```python
from build123d import *

# Parameters (mm, degrees)
BOSS_EXTRUDE2_DEPTH             = 400
SHELL3_T                        = -3
FILLET2_R                       = 50
FILLET3_R                       = 50
BOSS_EXTRUDE3_REACH             = 1052
SKETCH3_W                       = 40
SKETCH3_H                       = 40
BOSS_EXTRUDE3_DIRECTION_2_DEPTH = 19.71
SKETCH4_R                       = 7.5
CUT_EXTRUDE1_DEPTH              = 20


with BuildPart() as part:
    # Sketch2 → Boss-Extrude2 (new body)
    with BuildSketch(Plane.XY):
        Polygon((0, 400), (0, 0), (-400, 107.179676972), (-400, 207.179676972), align=None)
    extrude(amount=BOSS_EXTRUDE2_DEPTH)

    # Shell3
    shell3_openings = [part.faces().sort_by_distance(p)[0] for p in [
        (-400, 157.179676972, 200),
        (-200, 303.589838486, 200),
    ]]
    offset(amount=SHELL3_T, openings=shell3_openings, kind=Kind.INTERSECTION)

    # Fillet2
    fillet2_edges = [part.edges().sort_by_distance(p)[0] for p in [
        (-400, 207.179676972, 398.5),
    ]]
    fillet(fillet2_edges, radius=FILLET2_R)

    # Fillet3
    fillet3_edges = [part.edges().sort_by_distance(p)[0] for p in [
        (-400, 207.179676972, 1.5),
    ]]
    fillet(fillet3_edges, radius=FILLET3_R)

    # Sketch3 → Boss-Extrude3 (add, up to next)
    with BuildSketch(Plane(origin=(0, -650, 0), x_dir=(1, 0, 0), z_dir=(0, 1, 0)), mode=Mode.PRIVATE) as boss_extrude3_sk1:
        with Locations((-83, -60)):
            Rectangle(SKETCH3_W, SKETCH3_H)
    boss_extrude3_tool1 = extrude(boss_extrude3_sk1.sketch, amount=BOSS_EXTRUDE3_REACH, mode=Mode.PRIVATE) - part.part
    add(boss_extrude3_tool1.solids().sort_by_distance((-83, -650, 60))[0])
    # Sketch3 → Boss-Extrude3 (add, up to next)
    with BuildSketch(Plane(origin=(0, -650, 0), x_dir=(1, 0, 0), z_dir=(0, 1, 0)), mode=Mode.PRIVATE) as boss_extrude3_sk2:
        with Locations((-320, -60)):
            Rectangle(SKETCH3_W, SKETCH3_H)
    boss_extrude3_tool2 = extrude(boss_extrude3_sk2.sketch, amount=BOSS_EXTRUDE3_REACH, mode=Mode.PRIVATE) - part.part
    add(boss_extrude3_tool2.solids().sort_by_distance((-320, -650, 60))[0])
    # Sketch3 → Boss-Extrude3 (add, up to next)
    with BuildSketch(Plane(origin=(0, -650, 0), x_dir=(1, 0, 0), z_dir=(0, 1, 0)), mode=Mode.PRIVATE) as boss_extrude3_sk3:
        with Locations((-83, -340)):
            Rectangle(SKETCH3_W, SKETCH3_H)
    boss_extrude3_tool3 = extrude(boss_extrude3_sk3.sketch, amount=BOSS_EXTRUDE3_REACH, mode=Mode.PRIVATE) - part.part
    add(boss_extrude3_tool3.solids().sort_by_distance((-83, -650, 340))[0])
    # Sketch3 → Boss-Extrude3 (add, up to next)
    with BuildSketch(Plane(origin=(0, -650, 0), x_dir=(1, 0, 0), z_dir=(0, 1, 0)), mode=Mode.PRIVATE) as boss_extrude3_sk4:
        with Locations((-320, -340)):
            Rectangle(SKETCH3_W, SKETCH3_H)
    boss_extrude3_tool4 = extrude(boss_extrude3_sk4.sketch, amount=BOSS_EXTRUDE3_REACH, mode=Mode.PRIVATE) - part.part
    add(boss_extrude3_tool4.solids().sort_by_distance((-320, -650, 340))[0])

    # Sketch3 → Boss-Extrude3 direction 2 (add)
    with BuildSketch(Plane(origin=(0, -650, 0), x_dir=(1, 0, 0), z_dir=(0, 1, 0))):
        with Locations((-83, -60)):
            Rectangle(SKETCH3_W, SKETCH3_H)
        with Locations((-320, -60)):
            Rectangle(SKETCH3_W, SKETCH3_H)
        with Locations((-83, -340)):
            Rectangle(SKETCH3_W, SKETCH3_H)
        with Locations((-320, -340)):
            Rectangle(SKETCH3_W, SKETCH3_H)
    extrude(amount=-BOSS_EXTRUDE3_DIRECTION_2_DEPTH)

    # Sketch4 → Cut-Extrude1 (cut)
    with BuildSketch(Plane.XZ.offset(669.71)):
        with Locations((-320, 340)):
            Circle(SKETCH4_R)
        with Locations((-83, 340)):
            Circle(SKETCH4_R)
        with Locations((-320, 60)):
            Circle(SKETCH4_R)
        with Locations((-83, 60)):
            Circle(SKETCH4_R)
    extrude(amount=-CUT_EXTRUDE1_DEPTH, mode=Mode.SUBTRACT)


solid = part.part
```
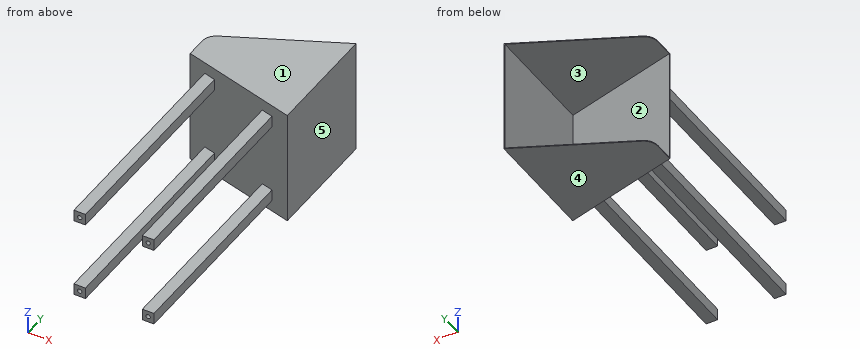
Work out the finished part from the listing and answer in its coordinate system (mm). Face numbers are marked on the shaded views. A direction names the side the tool comes from. Give positions to 0.01 mm unless a question says otherwise; leave off trailing zeros. Loops run counter-clockwise (first coordinate to the right, second up) from the corner with the lowest first, then second, coordinate; pieces in that order, holes last. Notation, with made-up numbers: (-11, 35.25) -> (3, 35.25) arc R16 ccw to (3, 64.25) -> close; hole circle Ø8 at (-34.5, 61). An arc over 180 degrees is marked (long way). Write item = value, one per line. Start each with the question number.
(1) Find section A-A on y = -397.5. Give the vertices of the cut face in (x, z).
(2) Find the intervals of material crossed by probe 1 along Z at (x, y) = (-320, -661); probe 2 along X at (y, z) = (-661.75, 340); probe 3 along X at (y, z) = (-619, 327), in increasing order. Write a range as from..to.
(3) Which of the six approach directions +Z, -Z, +X, -X, +Y, -Y give full straight-line access (tool end or side, diameter ignored) to the marked faces 1 and 2?
(4) The mould has two halves that part along X. Classify the marked faces 3, 4 and 5: +X half, -X half, draft (parallel to the pull), parting line (faces both ways), or undercut.
(5) Find section B-B on y = 149. Give the vertices of the cut face in (x, z).
(6) Given pin 1 Ø20 at (x, y) = (-314.5, -342.5) entering from -Z; pin 2 Ø1.5 at (x, z) = (-331.5, 356) entering from +Y; pin 3 Ø20 at (y, z) = (-246, 68.5) entering from -X, each flat-ended and moving along its own axis, determine where each tip first touches the part or whether it passes through.
(7) Find section C-C on x = -351. Give the vertices of the cut face in (y, z), and give its area (3 significant figures).
From the geometry:
q1.outline = (-340, 40) -> (-300, 40) -> (-300, 80) -> (-340, 80) -> close; (-340, 320) -> (-300, 320) -> (-300, 360) -> (-340, 360) -> close; (-103, 40) -> (-63, 40) -> (-63, 80) -> (-103, 80) -> close; (-103, 320) -> (-63, 320) -> (-63, 360) -> (-103, 360) -> close
q2.probe_1 = 40..52.5, 67.5..80, 320..332.5, 347.5..360
q2.probe_2 = -340..-327.5, -312.5..-300, -103..-90.5, -75.5..-63
q2.probe_3 = -340..-300, -103..-63
q3.face_1 = +Z, +X, -X, +Y, -Y
q3.face_2 = +Y
q4.face_3 = undercut
q4.face_4 = draft
q4.face_5 = +X half
q5.outline = (-400, 0) -> (0, 0) -> (0, 400) -> (-400, 400) -> (-400, 397) -> (-3, 397) -> (-3, 3) -> (-400, 3) -> close
q6.pin_1 = 40
q6.pin_2 = 92.13
q6.pin_3 = -340
q7.outline = (94.05, 0) -> (230.8, 0) -> (230.8, 3) -> (97.16, 3) -> (97.16, 397) -> (230.8, 397) -> (230.8, 400) -> (94.05, 400) -> close
q7.area = 2,040 mm^2
